```python
from build123d import *

# Parameters (mm, degrees)
SALIENTE_EXTRUIR4_DEPTH = 198
CROQUIS2_W              = 122.5
CROQUIS2_H              = 3
SALIENTE_EXTRUIR5_DEPTH = 13.963851332
CROQUIS3_R              = 5
CORTAR_EXTRUIR1_DEPTH   = 10
CHAFL_N2_SIZE           = 2


with BuildPart() as part:
    # Croquis1 → Saliente-Extruir4 (new body)
    with BuildSketch(Plane(origin=(0, 0, 0), x_dir=(1, 0, 0), z_dir=(0, 1, 0))):
        Polygon((-4, 10), (-4, 19.5), (7.5, 19.5), (7.5, 5.536148668), (130, 5.536148668), (130, 19.5), (141.5, 19.5), (141.5, 10), (137.5, 10), (137.5, 0), (0, 0), (0, 10), align=None)
    extrude(amount=SALIENTE_EXTRUIR4_DEPTH)

    # Croquis2 → Saliente-Extruir5 (add)
    with BuildSketch(Plane(origin=(0, 0, -5.536148668), x_dir=(-1, 0, 0), z_dir=(0, 0, -1))):
        with Locations((-68.75, 106.5)):
            Rectangle(CROQUIS2_W, CROQUIS2_H)
    extrude(amount=SALIENTE_EXTRUIR5_DEPTH)

    # Croquis3 → Cortar-Extruir1 (cut)
    with BuildSketch(Plane.XY):
        with Locations((68.75, 157.45296568)):
            Circle(CROQUIS3_R)
    extrude(amount=-CORTAR_EXTRUIR1_DEPTH, mode=Mode.SUBTRACT)

    # Chaflán2
    chafl_n2_edges = [part.edges().sort_by_distance(p)[0] for p in [
        (63.75, 157.45296568, -5.536148668),
    ]]
    chamfer(chafl_n2_edges, length=CHAFL_N2_SIZE)


solid = part.part
```
Here's how the part is built. I have some questions about the finished solid (model axes, mm). A direction names the side the tool comes from. Round coordinates to 2 decimals unless told otherwise and drop trailing zeros. Loops run counter-clockwise (first coordinate to the right, second up) from the corner with the lowest first, then second, coordinate; pieces in that order, holes last.
1. Will these pins go through, and if not, where does the flat tip stop? pin 1 (3 mm diameter, centred on y = 131, z = -2.5, fed in from +X); pin 2 (5 mm diameter, centred on y = 95.5, z = -6, fed in from -X); pin 3 (4 mm diameter, centred on x = 57.5, z = -13, fed in from +Y); pin 4 (6 mm diameter, centred on x = 68.75, y = 157.45, fed in from +Z).
Answers:
pin 1: stops at x = 137.5
pin 2: stops at x = 0
pin 3: stops at y = 108
pin 4: passes through
2. If I drill on probe 1 along X at (y, z) = (141, -10.25); probe 2 along Y at (x, z) = (68.75, -1.75); probe 3 along X at (y, z) = (78, -7.25), over which ranges is the centre line in solid material (lowest first)?
Answers:
probe 1: x = -4 to 7.5, 130 to 141.5
probe 2: y = 0 to 152.45, 162.45 to 198
probe 3: x = 0 to 7.5, 130 to 137.5
3. Suppose I cut it at A-A, the plane x = 68.75. Please give me the cut outline in (y, z).
Answers:
outline: (0, -5.54) - (105, -5.54) - (105, -19.5) - (108, -19.5) - (108, -5.54) - (150.45, -5.54) - (152.45, -3.54) - (152.45, 0) - (0, 0) - close; (162.45, -3.54) - (164.45, -5.54) - (198, -5.54) - (198, 0) - (162.45, 0) - close
4. Suppose I cut it at B-B, the plane x = 89. Please give me the cut outline in (y, z).
Answers:
outline: (0, -5.54) - (105, -5.54) - (105, -19.5) - (108, -19.5) - (108, -5.54) - (198, -5.54) - (198, 0) - (0, 0) - close
5. Suppose I cut it at D-D, the plane y = 110. Please give me the cut outline in (x, z).
Answers:
outline: (-4, -19.5) - (7.5, -19.5) - (7.5, -5.54) - (130, -5.54) - (130, -19.5) - (141.5, -19.5) - (141.5, -10) - (137.5, -10) - (137.5, 0) - (0, 0) - (0, -10) - (-4, -10) - close
6. Suppose I cut it at C-C, the plane z = -17.25. Please give me the cut outline in (x, y), and give its area (3 significant figures).
Answers:
outline: (-4, 0) - (7.5, 0) - (7.5, 105) - (130, 105) - (130, 0) - (141.5, 0) - (141.5, 198) - (130, 198) - (130, 108) - (7.5, 108) - (7.5, 198) - (-4, 198) - close
area: 4,920 mm2
7. For faces 4 (the face through (7.5, 52, -13)), 5 (the face through (140, 98, -10)), 6 (the face through (-2, 98, -10)), which set-ups out of +Z, -Z, +X, -X, +Y, -Y let a thin tool reach every point of the face, with its end or its side?
Answers:
face 4: -Z, -Y
face 5: +Z, +X, +Y, -Y
face 6: +Z, -X, +Y, -Y
8. Thinking about a two-plate mould opening in Y: for faces 1 (the face through (7.5, 152, -13)), 2 (the face through (70, 108, -12)), 3 (the face through (68.1, 162.41, -1.74)), which applies, released by +Y, released by -Y, zero draft, split by the parting line, or undercut?
Answers:
face 1: zero draft
face 2: released by +Y
face 3: undercut
